Design review of the part built by this model. Coordinates are the model's own, in mm. Give positions to 0.01 mm unless a question says otherwise; leave off trailing zeros. Loops run counter-clockwise (first coordinate to the right, second up) from the corner with the lowest first, then second, coordinate; pieces in that order, holes last. Notation, with made-up numbers: (27.25, 50.5) -> (40.25, 50.5) arc R26 cw to (40.25, 68.5) -> close; hole circle Ø7 at (12, 1.25). An arc over 180 degrees is marked (long way). Answer in a Markdown table with one row per item. Add a question column.
(1) Consider section A-A on x = 0. Write out the cut boundary in (y, z).
(2) Consider section D-D on y = 56. Write out the cut boundary in (x, z).
(3) Consider section B-B on y = -72. Write out the cut boundary in (x, z).
(4) For line 1 (X direction, y = -57.5, z = 0.7); line 2 (Y direction, x = -73, z = 0.4); line 3 (Y direction, x = 6.5, z = 3.9), list the stretches that pass through material, from the lowest coordinate up.
(5) Consider section C-C on x = 63.5. Write out the cut boundary in (y, z), then the cut area to 3 significant figures.
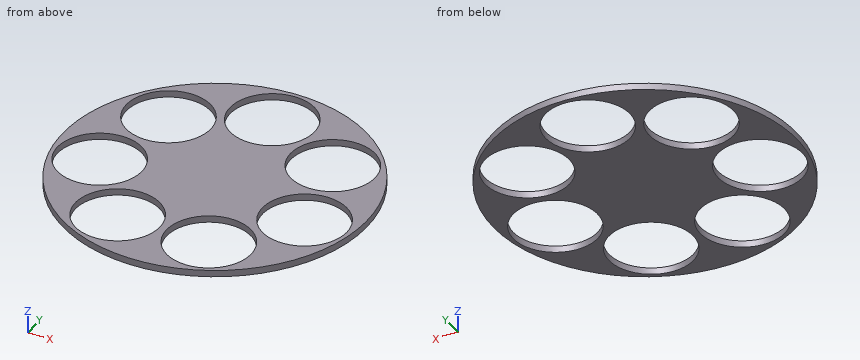
from build123d import *

# Parameters (mm, degrees)
F0_R            = 115
F1_DEPTH        = 5
F2_R            = 32
F3_DEPTH        = 5
F3_COPIES_COUNT = 7


# Not quite as in the source:
# - a pattern or mirror of a feature is missing from the dataset's text; its kind, count and spacing are read off the source's solid


with BuildPart() as f1:
    # F0 (on Top) → F1 (new body)
    with BuildSketch(Plane.XY):
        Circle(F0_R)
    extrude(amount=F1_DEPTH)

    # F2 (on face) → F3 (cut)
    with BuildSketch(Plane.XY.offset(5)):
        with Locations((0, 80)):
            Circle(F2_R)
    f3 = extrude(amount=-F3_DEPTH, mode=Mode.SUBTRACT)

    # F3_copies: F3 ×7 about axis
    f3_copies_axis = Axis((0, 0, 0), (0, 0, 1))
    for i in range(1, F3_COPIES_COUNT):
        add(f3.rotate(f3_copies_axis, i * 360 / F3_COPIES_COUNT), mode=Mode.SUBTRACT)


solid = f1.part
Values follow:
| question | item | result |
|---|---|---|
| 1 | outline | (-115, 0) -> (48, 0) -> (48, 5) -> (-115, 5) -> close; (112, 0) -> (115, 0) -> (115, 5) -> (112, 5) -> close |
| 2 | outline | (-100.44, 0) -> (-93.96, 0) -> (-93.96, 5) -> (-100.44, 5) -> close; (-31.14, 0) -> (-21.17, 0) -> (-21.17, 5) -> (-31.14, 5) -> close; (21.17, 0) -> (31.14, 0) -> (31.14, 5) -> (21.17, 5) -> close; (93.96, 0) -> (100.44, 0) -> (100.44, 5) -> (93.96, 5) -> close |
| 3 | outline | (-89.67, 0) -> (-66.71, 0) -> (-66.71, 5) -> (-89.67, 5) -> close; (-2.71, 0) -> (2.71, 0) -> (2.71, 5) -> (-2.71, 5) -> close; (66.71, 0) -> (89.67, 0) -> (89.67, 5) -> (66.71, 5) -> close |
| 4 | line 1 | -99.59 to -63.2, -6.22 to 6.22, 63.2 to 99.59 |
| 4 | line 2 | -88.86 to -49.41, 13.81 to 19.63, 80.12 to 88.86 |
| 4 | line 3 | -114.82 to -87.18, -56.97 to 48.67, 111.33 to 114.82 |
| 5 | outline | (-95.88, 0) -> (-86.05, 0) -> (-86.05, 5) -> (-95.88, 5) -> close; (-58.11, 0) -> (-46.33, 0) -> (-46.33, 5) -> (-58.11, 5) -> close; (10.73, 0) -> (17.89, 0) -> (17.89, 5) -> (10.73, 5) -> close; (81.86, 0) -> (95.88, 0) -> (95.88, 5) -> (81.86, 5) -> close |
| 5 | area | 214 mm2 |
